Could you check a few things on this model? Use its own coordinates, in mm. A direction names the side the tool comes from. Round coordinates to 2 decimals unless told otherwise and drop trailing zeros. Write each loop counter-clockwise with the first axis right and the second up, starting at its lowest first coordinate (ties: lowest second). Pieces come first, ordered by that corner, then holes. Notation, with made-up numbers: M 79.25,-32 L 84.25,-32 A31 cw 84.25,-3 Z; hole C -6,24.25 d6. An arc over 180 degrees is marked long. One line per question, with ' | ' between items. Start each with the question number.
Autodesk Inventor part; units mm, degrees
ref_plane "Work Plane1" through (30, 0, 0) normal (0, -0.5, 0.866) x (1, 0, 0)
ref_plane "YZ Plane" through (0, 0, 0) normal (1, 0, 0) x (0, 1, 0)
ref_plane "XZ Plane" through (0, 0, 0) normal (0, 1, 0) x (-1, 0, 0)
sketch "Sketch1" plane through (0, 0, 0) normal (0, 0, 1) x (1, 0, 0)
  line L0 (0.0567, 0) -> (12, 0)
  line L1 (12, 0) -> (12, 1.5)
  line L2 (12, 1.5) -> (1, 1.5)
  line L3 (1, 1.5) -> (0.6933, 1.5)
  line L4 (0.6933, 1.5) -> (0, 1.5)
  line L5 (0, 1.5) -> (0, 2.85)
  line L6 (0, 2.85) -> (-1.65, 2.85)
  line L7 (-1.65, 2.85) -> (-1.65, 1.1547)
  line L8 (-1.65, 1.1547) -> (-0.61, 1.1547)
  line L9 (-0.61, 1.1547) -> (0.0567, 0)
  line L10 (-4.38, 0) -> (14.73, 0)
  line L11 (0, -0.57) -> (0, 3.42)
  line L12 (1, 1.5) -> (0, 1.5) construction
  dimension "d0" = 11
  dimension "d1" = 0.3067
  dimension "d2" = 1.65
  dimension "d3" = 1.04
  dimension "d4" = 60
  dimension "d5" = 3
  dimension "d6" = 3
  dimension "d7" = 2.3094
  dimension "d8" = 5.7
  dimension "d19" = 12
revolve "Body" add sketch "Sketch1" angle 360 about axis through (0.0567, 0, 0) along (1, 0, 0) contours L9 L11 L4 L3 L2 L1 L0 | L9 L8 L7 L6 L5 L11
sketch "Sketch2" plane through (-1.65, 0, 0) normal (-1, 0, 0) x (0, 0, 1)
  circle A0 centre (0, 0) radius 1.1547
  line L0 (0, -3.99) -> (0, 3.99)
  line L1 (-3.99, 0) -> (3.99, 0)
  line L2 (1.1547, 0) -> (0.5774, -1)
  line L3 (0.5774, -1) -> (-0.5774, -1)
  line L4 (-0.5774, -1) -> (-1.1547, 0)
  line L5 (-1.1547, 0) -> (-0.5774, 1)
  line L6 (-0.5774, 1) -> (0.5774, 1)
  line L7 (0.5774, 1) -> (1.1547, 0)
extrude "Slot" add sketch "Sketch2" against normal up to next contours L7 A0 | A0 L2 | L6 L0 A0 | A0 L0 L3 | L0 L6 A0 | A0 L3 L0 | L4 A0 | A0 L5
fillet "Fillet1" radius 1.27 1 edges at (-1.65, -2.85, 0)
thread "Thread"
chamfer "Chamfer1" distance 0.3067 distance2 0.3067 1 edges at (12, -1.5, 0) measured on face at (12, -0.6587, -0.1791)
fillet "Fillet2" radius 0.1 1 edges at (0, -1.5, 0)
ref_plane "Work Plane1" through (30, 0, 0) normal (0, -0.5, 0.866) x (1, 0, 0)
equation "\"d0\" = GEL"
equation "\"d1\" = GAL"
equation "\"d2\" = KOH"
equation "\"d3\" = INTI"
equation "\"d5\" = GD"
equation "\"d6\" = BDM"
equation "\"d7\" = 1.1547 * SW"
equation "\"d8\" = KOD"
equation "\"d19\" = NLG"
equation "\"d16\" = RR"
equation "\"d12\" = GEL"
equation "\"d14\" = -0.5 * SPD + 0.5 * GD"
equation "\"d15\" = GUL"
equation "\"d29\" = R"
equation "\"GD\" = NND"
equation "\"NLG\" = 12"
equation "\"GEL\" = 11"
equation "\"KOD\" = 5.7"
equation "\"KOH\" = 1.65"
equation "\"INTI\" = 1.04"
equation "\"GAL\" = 0.61345 * PTC"
equation "\"GUL\" = 0.61345 * PTC"
equation "\"BDM\" = NND"
equation "\"SW\" = 2"
equation "\"RR\" = 1.27"
equation "\"SPD\" = 2.38655"
equation "\"d28\" = R"
equation "\"R\" = 0.1"
equation "\"TOA\" = 30deg"
equation "\"THREADDIA\" = 3"
equation "\"KOD1\" = KOD - 2 * RR"
equation "\"PTC\" = 0.5"
equation "\"NND\" = 3"
equation "\"E0\" = 1.155 * SW"
equation "\"GD1\" = THREADDIA - 1.2269 * PTC"
properties part number "ANSI B18.3.4M - M3 x 0.5 x 12, FHSBHCSM" material "Steel, Mild"
1. If we mould it in two halves opening along Z, with no side actions, what happens to faces 1 (the face through (-1.09, -0.51, -0.86)), 2 (the face through (5.82, -1.5, -0.07)), 3 (the face through (0, 0, -2))? For each: released by +Z, released by -Z, zero draft, split by the parting line, or undercut.
2. Suppose I cut it at A-A (x = 3.75). Write out the boundary of the cut face in (y, z).
3. Which directions (+Z, -Z, +X, -X, +Y, -Y) give clear straight access to the entire face, cutting with the end or side of a thin tool? Please do faces 4 (the face through (-0.193, -2.262, 1.734)), 5 (the face through (-1.09, 0.49, -0.87)).
4. I'm going to push flat-ended pins straight in: P1, Ø0.9, axis at x = -1.5, z = 0, coming from the -Y side; P2, Ø1.5, axis at x = 9.5, y = 2, coming from the -Z side; P3, Ø2, axis at x = 10.5, y = 1.5, coming from the -Z side. Where does each tip first touch, or does it pass through?
5. I need wall thicknesses on line 1 along X through (y, z) = (1.3, -1.5); line 2 along Y through (x, z) = (-0.75, 0.05); line 3 along Z through (x, y) = (4.75, 0.25). Which ranges of each line are inside material? Lowest first, please. Write a range as from..to.
Computed:
1) face 1: undercut | face 2: split by the parting line | face 3: zero draft
2) outline: C 0,0 d3
3) face 4: +X, -X | face 5: -X
4) P1: stops at y = -2.66 | P2: stops at z = -0.83 | P3: stops at z = -1.41
5) line 1: x = -1.58..0 | line 2: y = -2.79..-1, 1..2.79 | line 3: z = -1.48..1.48
